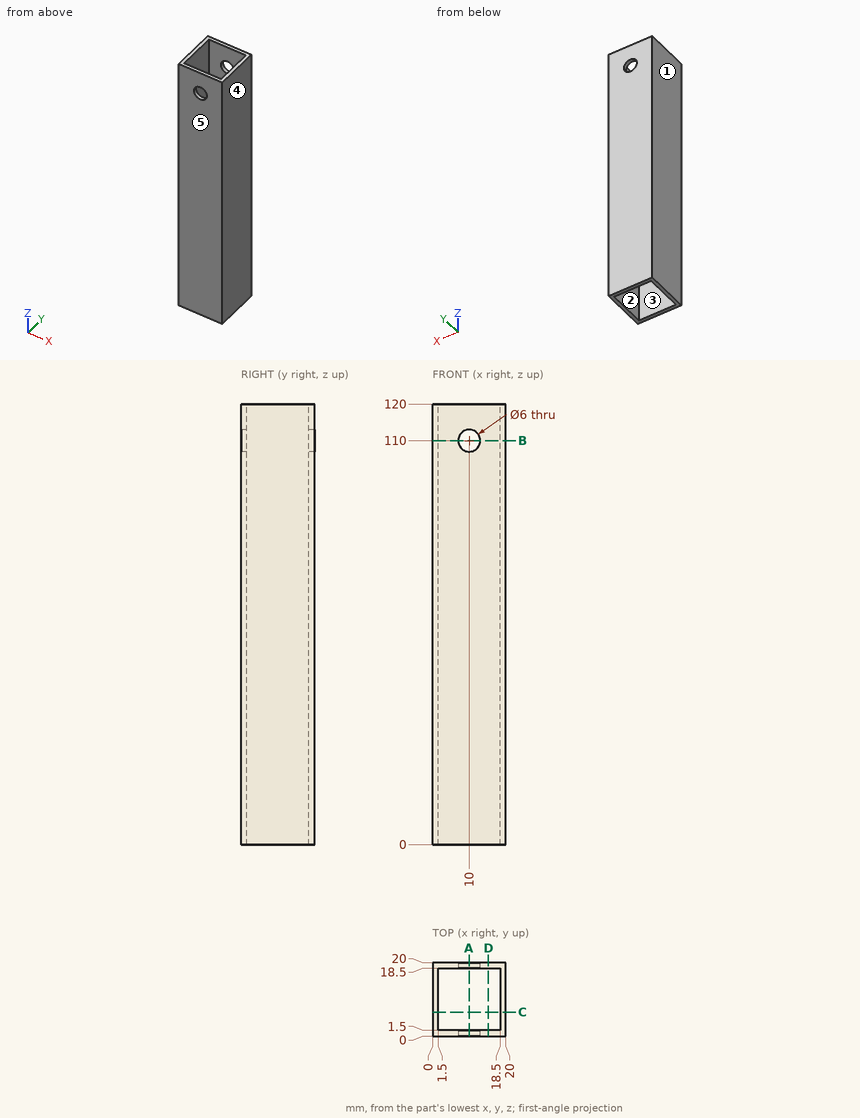
Answer from the drawing. Dimensions are ordinates in mm from the lowest x, y and z of the part. A direction names the side the tool comes from. Give positions to 0.01 mm unless a question says otherwise; leave off trailing zeros. Order: outer loops, then holes, each group sorted by start corner. A loop starts at its lowest first (then second) coordinate and runs counter-clockwise, first axis right, second up. Notation, with made-up numbers: (-31, -4.75) - (13, -4.75) arc R19 cw to (13, 17.25) - close; hole circle Ø4 at (-39.75, 25). An arc over 180 degrees is marked (long way). One line per item, written item: value. Start each with the question number.
1) A cutting plane is placed at C-C on y = 6.5. Give the vertices of the cut face in (x, z).
2) Find the intervals of material crossed by L1, parallel to X at y = 12, z = 73.5; L2, parallel to Z at x = 10, y = 19.45, in increasing order.
3) Given pin 1 Ø9.5 at (x, z) = (10, 110) entering from -Y; pin 2 Ø5 at (x, z) = (10, 110) entering from +Y, each flat-ended and moving along its own axis, determine where each tip first touches the part or whether it passes through.
4) A cutting plane is placed at A-A on x = 10. Give the vertices of the cut face in (y, z), then the cut area to 3 significant figures.
5) A cutting plane is placed at B-B on z = 110. Give the vertices of the cut face in (x, y).
6) A tool of negligible diameter and unlimited length cuts with its end or side. For the marked faces 1 and 2, from which of +Z, -Z, +X, -X, +Y, -Y can it reach the whole face along a straight path? Write none if from no direction.
7) The mould has two halves that part along X. Classify the marked faces 3, 4 and 5: released by +X, released by -X, zero draft, split by the parting line, or undercut.
Answer sheet:
1. outline: (0, 0) - (1.5, 0) - (1.5, 120) - (0, 120) - close; (18.5, 0) - (20, 0) - (20, 120) - (18.5, 120) - close
2. L1: x = 0 to 1.5, 18.5 to 20
2. L2: z = 0 to 107, 113 to 120
3. pin 1: stops at y = 0
3. pin 2: passes through
4. outline: (0, 0) - (1.5, 0) - (1.5, 107) - (0, 107) - close; (0, 113) - (1.5, 113) - (1.5, 120) - (0, 120) - close; (18.5, 0) - (20, 0) - (20, 107) - (18.5, 107) - close; (18.5, 113) - (20, 113) - (20, 120) - (18.5, 120) - close
4. area: 342 mm2
5. outline: (0, 0) - (7, 0) - (7, 1.5) - (1.5, 1.5) - (1.5, 18.5) - (7, 18.5) - (7, 20) - (0, 20) - close; (13, 0) - (20, 0) - (20, 20) - (13, 20) - (13, 18.5) - (18.5, 18.5) - (18.5, 1.5) - (13, 1.5) - close
6. face 1: +Z, -Z, -X, +Y, -Y
6. face 2: +Z, -Z
7. face 3: undercut
7. face 4: released by +X
7. face 5: zero draft
